Geometry check sheet. Reference: the model listing, model coordinates, mm. A direction names the side the tool comes from. Round coordinates to 2 decimals unless told otherwise and drop trailing zeros. Order: outer loops, then holes, each group sorted by start corner. A loop starts at its lowest first (then second) coordinate and runs counter-clockwise, first axis right, second up.
(1) Set-up check for faces 1 (the face through (-31.93, 27.07, -16.3)), 2 (the face through (-19.05, -26, 23)), 3 (the face through (-0.293, 1.907, 73.68)), 4 (the face through (19, -1, 54.541)), 5 (the face through (19.228, 25.8, -17.367)): record each of +Z, -Z, +X, -X, +Y, -Y from which the full face is reachable in a straight line by a thin tool's end or side.
(2) Gauge pin test, flat ends, axial feed: P1, Ø11.5, axis at y = -30.48, z = -21.66, coming from the +X side; P2, Ø8, axis at y = -30.5, z = 9.5, coming from the -X side; P3, Ø12, axis at y = -7.5, z = 7.5, coming from the -X side; P4, Ø1, axis at y = 25, z = 45, coming from the +X side. Record the tip position at first contact, or that the pin passes through.
(3) Cross-section at B-B on y = 0. Enter the section's corners in (x, z).
(4) Cross-section at C-C on x = 19.5. Enter the section's corners in (y, z), and give its area (3 significant figures).
(5) Cross-section at A-A on x = -6.35. Enter the section's corners in (y, z).
(6) Cross-section at D-D on y = -49. Enter the section's corners in (x, z).
(7) Thickness scan on L1, parallel to Z at x = 16.75, y = -30.48; L2, parallel to Z at x = 11.43, y = -47.25; L3, parallel to Z at x = 7, y = -12. Record the ranges inside material, lowest first.
(8) Draft check along X on faces 6 (the face through (-32, -1, 54.541)), 7 (the face through (-6, 0, 67.241)), 8 (the face through (-19.05, -30, -22)). Enter one of: pulls with the +X half, pulls with the -X half, needs draft (parallel to the pull), parting line crosses it, or undercut.
from build123d import *

# Parameters (mm, degrees)
F1_DEPTH  = 38.1
F3_D      = 50.8
F5_R      = 6.35
F6_DEPTH  = 25.4
F4_R      = 6.35
F7_DEPTH  = 25.4
F8_R      = 6.35
F9_DEPTH  = 12.7
F10_R     = 1
F10_R_2   = 0.746
F11_DEPTH = 25.4
F10_R_3   = 10.16
F12_DEPTH = 101.6


with BuildPart() as f1:
    # F0 (on Front) → F1 (new body, symmetric)
    with BuildSketch(Plane.XZ):
        Polygon((-44.45, -8.95857), (-44.45, -34.35857), (31.75, -34.35857), (31.75, -8.95857), (6.35, -8.95857), (6.35, 54.54143), (31.75, 54.54143), (31.75, 79.94143), (-44.45, 79.94143), (-44.45, 54.54143), (-19.05, 54.54143), (-19.05, -8.95857), align=None)
    extrude(amount=F1_DEPTH, both=True)

    # F3 (through all)
    with Locations(Plane.YZ.offset(6.35)):
        with Locations((0, 22.79143)):
            Hole(F3_D / 2)

    # F5 (on face) → F6 (cut)
    with BuildSketch(Plane.YZ.offset(31.75)):
        with Locations((-30.48, -21.65857)):
            Circle(F5_R)
        with Locations((30.48, -21.65857)):
            Circle(F5_R)
    extrude(amount=-F6_DEPTH, mode=Mode.SUBTRACT)

    # F4 (on face) → F7 (cut)
    with BuildSketch(Plane(origin=(-44.45, 0, 0), x_dir=(0, -1, 0), z_dir=(-1, 0, 0))):
        with Locations((30.48, -21.65857)):
            Circle(F4_R)
        with Locations((-30.48, -21.65857)):
            Circle(F4_R)
    extrude(amount=-F7_DEPTH, mode=Mode.SUBTRACT)

    # F8 (on face) → F9 (cut)
    with BuildSketch(Plane.XY.offset(79.94143)):
        with Locations((-6.35, 0)):
            Circle(F8_R)
    extrude(amount=-F9_DEPTH, mode=Mode.SUBTRACT)

    # F10 (on face) → F11 (join)
    with BuildSketch(Plane.XZ.offset(38.1)):
        with Locations((11.43, 59.62143)):
            Circle(F10_R)
        with Locations((11.43, 59.62143)):
            Circle(F10_R_2, mode=Mode.SUBTRACT)
        with Locations((-24.13, 59.62143)):
            Circle(F10_R)
        with Locations((-24.13, 59.62143)):
            Circle(F10_R_2, mode=Mode.SUBTRACT)
    extrude(amount=F11_DEPTH)

    # F10 (on face) → F12 (cut)
    with BuildSketch(Plane.XZ.offset(38.1)):
        with Locations((-6.35, 22.79143)):
            Circle(F10_R_3)
    extrude(amount=-F12_DEPTH, mode=Mode.SUBTRACT)


solid = f1.part
Found:
1. face 1: -X
1. face 2: -X, +Y, -Y
1. face 3: +Z
1. face 4: +X, +Y, -Y
1. face 5: +X
2. P1: stops at x = 6.35
2. P2: stops at x = -19.05
2. P3: passes through
2. P4: stops at x = 6.35
3. outline: (-44.45, -34.36) - (31.75, -34.36) - (31.75, -8.96) - (6.35, -8.96) - (6.35, -2.61) - (-19.05, -2.61) - (-19.05, -8.96) - (-44.45, -8.96) - close; (-44.45, 54.54) - (-19.05, 54.54) - (-19.05, 48.19) - (6.35, 48.19) - (6.35, 54.54) - (31.75, 54.54) - (31.75, 79.94) - (0, 79.94) - (0, 67.24) - (-12.7, 67.24) - (-12.7, 79.94) - (-44.45, 79.94) - close
4. outline: (-38.1, -34.36) - (38.1, -34.36) - (38.1, -8.96) - (-38.1, -8.96) - close; (-38.1, 54.54) - (38.1, 54.54) - (38.1, 79.94) - (-38.1, 79.94) - close; hole circle Ø12.7 at (-30.48, -21.66); hole circle Ø12.7 at (30.48, -21.66)
4. area: 3,620 mm2
5. outline: (-38.1, -34.36) - (38.1, -34.36) - (38.1, 12.63) - (23.28, 12.63) arc R25.4 cw to (-23.28, 12.63) - (-38.1, 12.63) - close; (-38.1, 32.95) - (-23.28, 32.95) arc R25.4 cw to (23.28, 32.95) - (38.1, 32.95) - (38.1, 79.94) - (6.35, 79.94) - (6.35, 67.24) - (-6.35, 67.24) - (-6.35, 79.94) - (-38.1, 79.94) - close
6. outline: circle Ø2 at (-24.13, 59.62); circle Ø2 at (11.43, 59.62); hole circle Ø1.49 at (-24.13, 59.62); hole circle Ø1.49 at (11.43, 59.62)
7. L1: z = -34.36 to -28.01, -15.31 to -8.96, 54.54 to 79.94
7. L2: z = 58.62 to 58.88, 60.37 to 60.62
7. L3: z = -34.36 to -8.96, 54.54 to 79.94
8. face 6: needs draft
8. face 7: undercut
8. face 8: pulls with the -X half
